```python
from build123d import *

# Parameters (mm, degrees)
F0_W           = 133.3499997854
F0_H           = 127
F0_R           = 3.175
F0_R_2         = 15.24
F1_DEPTH       = 19.05
F4_D           = 5.1054
F4_DEPTH       = 25.4
F4_TIP         = 1.5338169022
F4_ON_F3_D     = 5.1054
F4_ON_F3_DEPTH = 25.4
F4_ON_F3_TIP   = 1.5338169022
F7_R           = 12.7


with BuildPart() as f1:
    # F0 (on Front) → F1 (new body)
    with BuildSketch(Plane.XZ):
        with Locations((-66.6749998927, 63.5)):
            Rectangle(F0_W, F0_H)
        with Locations((-117.5500062, 41.1999938)):
            Circle(F0_R, mode=Mode.SUBTRACT)
        with Locations((-47.5499938, 41.1999938)):
            Circle(F0_R, mode=Mode.SUBTRACT)
        with Locations((-82.55, 76.2)):
            Circle(F0_R_2, mode=Mode.SUBTRACT)
        with Locations((-117.5500062, 111.2000062)):
            Circle(F0_R, mode=Mode.SUBTRACT)
        with Locations((-47.5499938, 111.2000062)):
            Circle(F0_R, mode=Mode.SUBTRACT)
    extrude(amount=F1_DEPTH)

    # F4
    with Locations(Plane.YZ):
        with Locations((-9.525, 101.6), (-9.525, 38.1)):
            Hole(F4_D / 2, depth=F4_DEPTH)
            with Locations((0, 0, -(F4_DEPTH + F4_TIP / 2))):  # 118° drill point
                Cone(0, F4_D / 2, F4_TIP, mode=Mode.SUBTRACT)

    # F4 on F3
    with Locations(Plane(origin=(0, 0, 0), x_dir=(1, 0, 0), z_dir=(0, 0, -1))):
        with Locations((-25.4, 9.525), (-88.9, 9.525)):
            Hole(F4_ON_F3_D / 2, depth=F4_ON_F3_DEPTH)
            with Locations((0, 0, -(F4_ON_F3_DEPTH + F4_ON_F3_TIP / 2))):  # 118° drill point
                Cone(0, F4_ON_F3_D / 2, F4_ON_F3_TIP, mode=Mode.SUBTRACT)


with BuildPart() as f5_1:
    # F5: instance of F1
    add(f1.part.mirror(Plane(origin=(-65.8295348944, -19.05, 62.823628006), x_dir=(1, 0, 0), z_dir=(0, -1, 0))))

    # F7
    f7_edges = [f5_1.edges().sort_by_distance(p)[0] for p in [
        (-133.35, -28.575, 127),
    ]]
    fillet(f7_edges, radius=F7_R)


solid = f5_1.part
```
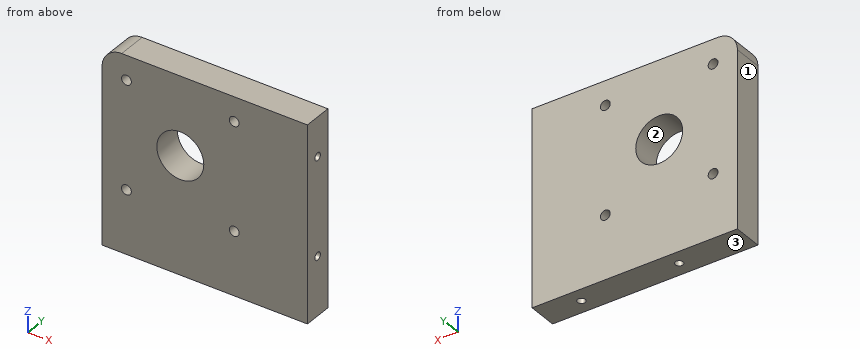
Geometry check sheet. Reference: the model listing, model coordinates, mm. Face numbers are marked on the shaded views. Coordinates: 2 decimals unless noted, no trailing zeros. Write each loop counter-clockwise with the first axis right and the second up, starting at its lowest first coordinate (ties: lowest second). Pieces come first, ordered by that corner, then holes. Notation, with made-up numbers: (-9.5, -30) -> (40.5, -30) arc R17 cw to (40.5, -19) -> close; hole circle Ø11 at (21.5, 35.25). An arc over 180 degrees is marked (long way). Use CSV: the item, a comma, the result in double quotes. Start each with the question number.
Item 1: Cross-section at A-A, the plane x = -82.55. Record the cut outline in (y, z), plus the area to 3 significant figures.
Item 2: Mould release check, pull along X, two halves, no side actions. Record for the marked faces 1, 2 and 3: released by +X, released by -X, zero draft, split by the parting line, or undercut.
Item 3: Cross-section at B-B, the plane z = 76.2. Record the cut outline in (x, y).
Item 4: Thickness scan on line 1 (X direction, y = -34.5, z = 41); line 2 (X direction, y = -26.25, z = 11); line 3 (Z direction, x = -81.5, y = -21.75). Record the ranges inside material, lowest first.
Item 5: Cross-section at C-C, the plane y = -22. Record the cut outline in (x, z) (3 decimals), plus the area to 3 significant figures.
Item 6: Depth check by flat-ended pin: pin 1 Ø4 at (x, y) = (-88.9, -28.575) entering from -Z. Enter the tip coordinate at first touch or a pass-through.
Answers:
1,outline,"(-38.1, 0) -> (-19.05, 0) -> (-19.05, 60.96) -> (-38.1, 60.96) -> close; (-38.1, 91.44) -> (-19.05, 91.44) -> (-19.05, 127) -> (-38.1, 127) -> close"
1,area,"1,840 mm^2"
2,face 1,"released by -X"
2,face 2,"undercut"
2,face 3,"zero draft"
3,outline,"(-133.35, -38.1) -> (-97.79, -38.1) -> (-97.79, -19.05) -> (-133.35, -19.05) -> close; (-67.31, -38.1) -> (0, -38.1) -> (0, -19.05) -> (-67.31, -19.05) -> close"
4,line 1,"-133.35 to -120.72, -114.38 to -50.72, -44.38 to 0"
4,line 2,"-133.35 to -89.95, -87.85 to -26.45, -24.35 to 0"
4,line 3,"0 to 61, 91.4 to 127"
5,outline,"(-133.35, 0) -> (0, 0) -> (0, 127) -> (-120.65, 127) arc R12.7 ccw to (-133.35, 114.3) -> close; hole circle Ø6.35 at (-117.55, 41.2); hole circle Ø6.35 at (-117.55, 111.2); hole circle Ø30.48 at (-82.55, 76.2); hole circle Ø6.35 at (-47.55, 41.2); hole circle Ø6.35 at (-47.55, 111.2)"
5,area,"16,000 mm^2"
6,pin 1,"z = 25.73"
